Design review of the part built by this model. Coordinates are the model's own, in mm. Face numbers are marked on the shaded views. A direction names the side the tool comes from. Coordinates: 2 decimals unless noted, no trailing zeros. Write each loop counter-clockwise with the first axis right and the second up, starting at its lowest first coordinate (ties: lowest second). Pieces come first, ordered by that corner, then holes. Notation, with made-up numbers: (75, 75.25) - (89, 75.25) arc R25 cw to (89, 97.25) - close; hole circle Ø10 at (1.25, 41.25). An arc over 180 degrees is marked (long way). Answer as a JSON object with one key per item and string values.
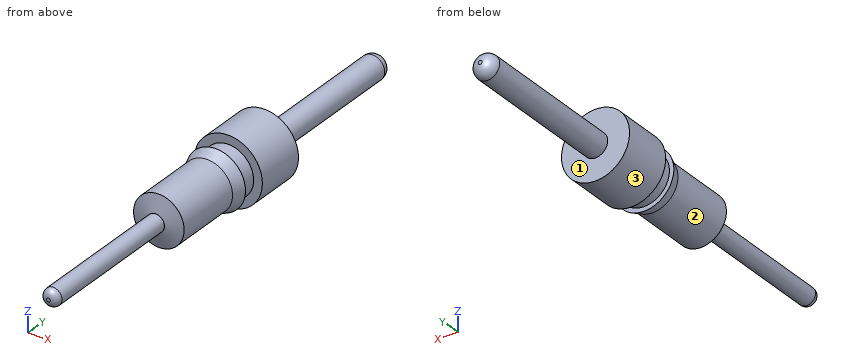
Autodesk Inventor part; units mm, degrees
ref_plane "pins_XY" through (0, 0, 0) normal (0, 1, 0) x (1, 0, 0)
ref_plane "pins_YZ" through (0, 0, 0) normal (1, 0, 0) x (0, 0, -1)
ref_plane "pins_ZX" through (0, 0, 0) normal (0, 0, -1) x (0, 1, 0)
sketch "Sketch_1" plane through (0, 0, 0) normal (0, 0, 1) x (1, 0, 0)
  line L0 (0, -2.717) -> (0, 1.3208)
  line L1 (0, 1.3208) -> (0.889, 1.3208)
  line L2 (0.889, 1.3208) -> (0.889, 0)
  line L3 (0.889, 0) -> (0.6604, 0)
  line L4 (0.6604, 0) -> (0.6604, -0.4572)
  line L5 (0.6604, -0.4572) -> (0.7747, -0.4572)
  line L6 (0.7747, -0.4572) -> (0.6604, -0.7712)
  line L7 (0.6604, -0.7712) -> (0.6604, -2.54)
  line L8 (0.6604, -2.54) -> (0, -2.717)
  line L9 (0, -2.717) -> (0, 1.3208)
revolve "Revolution1" add sketch "Sketch_1" angle 360 about axis through (0, -2.717, 0) along (0, -1, 0)
sketch "Sketch_3" plane through (0, 0, 0) normal (0, 0, 1) x (1, 0, 0)
  line L0 (0, 1.3208) -> (0, 5.5372)
  line L1 (0, 5.5372) -> (0.0508, 5.5372)
  arc A0 (0.3175, 5.2705) -> (0.0508, 5.5372) centre (0.0508, 5.2705) ccw
  line L2 (0.3175, 5.2705) -> (0.3175, 1.3208)
  line L3 (0.3175, 1.3208) -> (0, 1.3208)
  line L4 (0, 1.3208) -> (0, 5.5372)
revolve "Revolution2" add sketch "Sketch_3" angle 360 about axis through (0, 1.3208, 0) along (0, -1, 0)
sketch "Sketch_14" plane through (0, 0, 0) normal (0, 0, 1) x (1, 0, 0)
  line L0 (0, -6.5786) -> (0, -1.6256)
  line L1 (0, -1.6256) -> (0.2286, -1.6256)
  line L2 (0.2286, -1.6256) -> (0.2286, -6.4008)
  arc A0 (0.0508, -6.5786) -> (0.2286, -6.4008) centre (0.0508, -6.4008) ccw
  line L3 (0.0508, -6.5786) -> (0, -6.5786)
  line L4 (0, -6.5786) -> (0, -1.6256)
revolve "Revolution3" add sketch "Sketch_14" angle 360 about axis through (0, -6.5786, 0) along (0, -1, 0)
ref_plane "pins_XY" through (0, 0, 0) normal (0, 1, 0) x (1, 0, 0)
ref_plane "pins_YZ" through (0, 0, 0) normal (1, 0, 0) x (0, 0, -1)
ref_plane "pins_ZX" through (0, 0, 0) normal (0, 0, -1) x (0, 1, 0)
properties part number "-101-G-A_pins"
(1) To check wall thickness, follow line 1 (Y direction, x = 0.55, z = -0.6); line 2 (Z direction, x = 0.05, y = -1.75); line 3 (Y direction, x = -0.6, z = 0.35). State the ranges of each line that lie inside material, in increasing order. Write a range as from..to.
Solved:
{"line 1": "y = 0..1.32", "line 2": "z = -0.66..0.66", "line 3": "y = -0.68..-0.46, 0..1.32"}
(2) Tool access review of the marked faces 1, 2 and 3: name each direction out of +Z, -Z, +X, -X, +Y, -Y from which nothing blocks a thin tool from reaching the whole face with its end or side.
Solved:
{"face 1": "+Y", "face 2": "-Y", "face 3": "+Y, -Y"}
(3) For pin 1 (0.5 mm diameter, centred on x = -0.5, z = -0.5, fed in from -Y); pin 2 (1 mm diameter, centred on x = -0.5, y = -2.5, fed in from +Z), all flat-tipped, find the tip position at first contact; note any pin that passes through.
Solved:
{"pin 1": "stops at y = -2.59", "pin 2": "stops at z = 0.66"}
(4) Take a section at B-B, the plane y = 4.25. Write out the cut boundary in (x, z) (1 decimal).
Solved:
{"outline": "circle Ø0.6 at (0, 0)"}
(5) Take a section at A-A, the plane y = -5.5. Write out the cut boundary in (x, z), and give its area (3 significant figures).
Solved:
{"outline": "circle Ø0.46 at (0, 0)", "area": "0.164 mm^2"}
